Design review of the part built by this model. Coordinates are the model's own, in mm. Face numbers are marked on the shaded views. A direction names the side the tool comes from. Give positions to 0.01 mm unless a question says otherwise; leave off trailing zeros. Loops run counter-clockwise (first coordinate to the right, second up) from the corner with the lowest first, then second, coordinate; pieces in that order, holes last. Notation, with made-up numbers: (-16, 34) -> (41, 34) arc R23 ccw to (41, 51) -> close; hole circle Ø7 at (24, -18). An arc over 180 degrees is marked (long way). Answer in a Markdown table with one row per item. Add a question column.
(1) Consider section A-A on x = 4. Write out the cut boundary in (y, z) (3 decimals).
(2) For pin 1 (17.5 mm diameter, centred on y = 28, z = -22.5, fed in from -X); pin 2 (1.5 mm diameter, centred on y = 29.5, z = -4.5, fed in from +X); pin 3 (10 mm diameter, centred on y = 7.5, z = -18.5, fed in from +X); pin 4 (2 mm diameter, centred on x = 2, z = -12, fed in from +Y), all flat-tipped, find the tip position at first contact; note any pin that passes through.
(3) Consider section B-B on y = 19.05. Count the separate pieces of the cut face and the enclosed holes in it, then the cut area to 3 significant figures.
(4) For line 1 (X direction, y = 26, z = -27) (3 decimals); line 2 (X direction, y = 24, z = 0) (3 decimals); line 3 (Z direction, x = -12, y = 28.5), list the stretches that pass through material, from the lowest coordinate up.
(5) For the marked faces 1 and 2, list the 3-axis set-ups (+Z, -Z, +X, -X, +Y, -Y) from which the entire face can be reached by the end or side of a thin tool; tool diameter is ignored.
(6) Consider section C-C on z = 0. Write out the cut boundary in (x, y) (3 decimals).
(7) Draft analysis for pull direction X (two halves, no side actions). For the marked faces 3, 4, 5 and 6, state which applies: +X half, -X half, draft (parallel to the pull), parting line (faces both ways), or undercut.
from build123d import *

# Parameters (mm, degrees)
SKETCH1_R           = 16.764
SKETCH1_R_2         = 13.335
BOSS_EXTRUDE1_DEPTH = 38.1
SKETCH2_W           = 6.35
SKETCH2_H           = 3.812490435
CUT_EXTRUDE1_DEPTH  = 45.873972322
SKETCH3_W           = 3.175
SKETCH3_H           = 19.05
BOSS_EXTRUDE2_DEPTH = 38.1
SKETCH4_R           = 3.175
CUT_EXTRUDE2_DEPTH  = 57.396744492


with BuildPart() as part:
    # Sketch1 → Boss-Extrude1 (new body)
    with BuildSketch(Plane(origin=(0, 0, 0), x_dir=(1, 0, 0), z_dir=(0, 1, 0))):
        with Locations(Location((0, 0, 0), (0, 0, 90))):
            Circle(SKETCH1_R)
        with Locations(Location((0, 0, 0), (0, 0, 90))):
            Circle(SKETCH1_R_2, mode=Mode.SUBTRACT)
    extrude(amount=BOSS_EXTRUDE1_DEPTH)

    # Sketch2 → Cut-Extrude1 (cut, through all)
    with BuildSketch(Plane(origin=(0, 38.1, 0), x_dir=(1, 0, 0), z_dir=(0, 1, 0))):
        with Locations((0, 14.857754782)):
            Rectangle(SKETCH2_W, SKETCH2_H)
    extrude(amount=-CUT_EXTRUDE1_DEPTH, mode=Mode.SUBTRACT)

    # Sketch3 → Boss-Extrude2 (add)
    with BuildSketch(Plane(origin=(0, 38.1, 0), x_dir=(1, 0, 0), z_dir=(0, 1, 0))):
        with Locations((-4.7625, 25.039805703)):
            Rectangle(SKETCH3_W, SKETCH3_H)
    boss_extrude2 = extrude(amount=-BOSS_EXTRUDE2_DEPTH)

    # Sketch4 → Cut-Extrude2 (cut, through all)
    with BuildSketch(Plane.ZY.offset(6.35)):
        with Locations((-25.039805703, 19.05)):
            Circle(SKETCH4_R)
    cut_extrude2 = extrude(amount=-CUT_EXTRUDE2_DEPTH, mode=Mode.SUBTRACT)

    # Mirror1: Boss-Extrude2, Cut-Extrude2 across plane
    add(boss_extrude2.mirror(Plane(origin=(0, 0, 0), x_dir=(0, 0, 1), z_dir=(1, 0, 0))))
    add(cut_extrude2.mirror(Plane(origin=(0, 0, 0), x_dir=(0, 0, 1), z_dir=(1, 0, 0))), mode=Mode.SUBTRACT)


solid = part.part
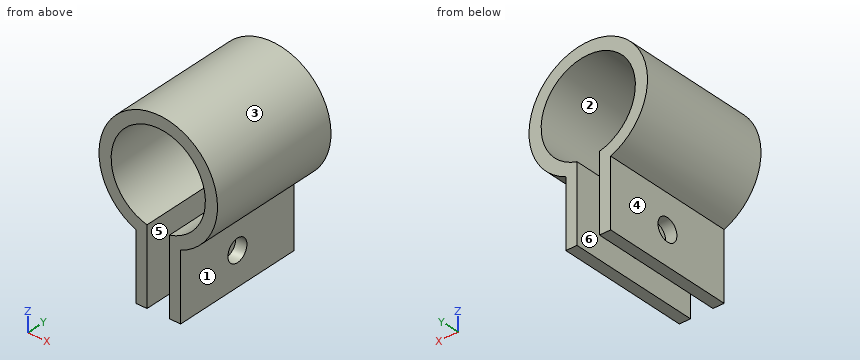
Values follow:
| question | item | result |
|---|---|---|
| 1 | outline | (0, -34.565) -> (38.1, -34.565) -> (38.1, -12.721) -> (0, -12.721) -> close; (0, 12.721) -> (38.1, 12.721) -> (38.1, 16.28) -> (0, 16.28) -> close; hole circle Ø6.35 at (19.05, -25.04) |
| 2 | pin 1 | x = -9.59 |
| 2 | pin 2 | x = 16.34 |
| 2 | pin 3 | x = 9.94 |
| 2 | pin 4 | through |
| 3 | separate pieces | 3 |
| 3 | enclosed holes | 0 |
| 3 | area | 380 mm2 |
| 4 | line 1 | -6.35 to -3.175, 3.175 to 6.35 |
| 4 | line 2 | -16.764 to -13.335, 13.335 to 16.764 |
| 4 | line 3 | -11.71 to -5.82, 5.82 to 11.71 |
| 5 | face 1 | -Z, +X, +Y, -Y |
| 5 | face 2 | +Y, -Y |
| 6 | outline | (-16.764, 0) -> (-13.335, 0) -> (-13.335, 38.1) -> (-16.764, 38.1) -> close; (13.335, 0) -> (16.764, 0) -> (16.764, 38.1) -> (13.335, 38.1) -> close |
| 7 | face 3 | parting line |
| 7 | face 4 | -X half |
| 7 | face 5 | undercut |
| 7 | face 6 | undercut |
